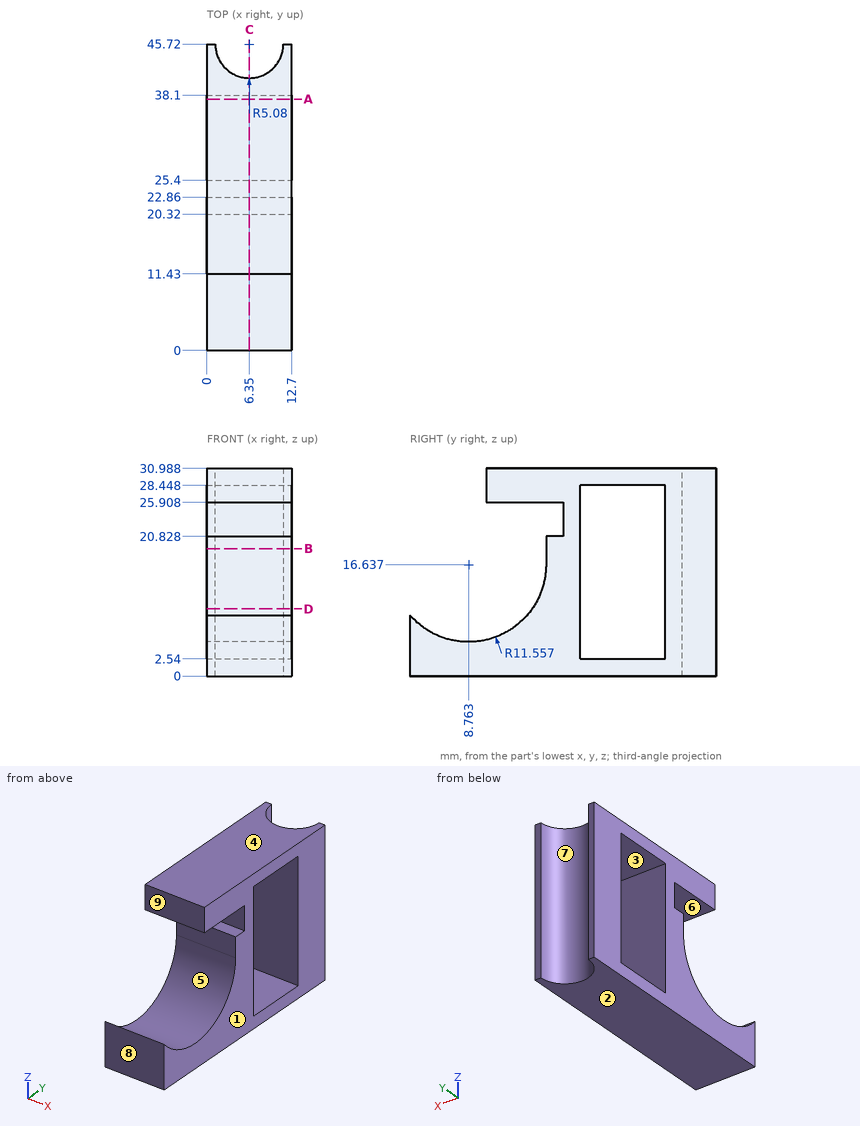
For this review, use the dimensioned drawing (mm, ordinates from the lowest corner) and the shaded views. A direction names the side the tool comes from. Give positions to 0.01 mm unless a question says otherwise; leave off trailing zeros. Order: outer loops, then holes, each group sorted by start corner. A loop starts at its lowest first (then second) coordinate and runs counter-clockwise, first axis right, second up.
1) Wall thickness on line 1 (Z direction, x = 6.25, y = 30); line 2 (Y direction, x = 3, z = 6); line 3 (Z direction, x = 1, y = 19): over which ranges is each line inside the solid? List them lowest first.
2) Take a section at D-D (z = 10). Give the boundary of the cut face in (x, y), then the cut area to 3 significant figures.
3) Take a section at C-C (x = 6.35). Give the boundary of the cut face in (y, z), then the cut area to 3 significant figures.
4) Take a section at B-B (z = 19). Give the boundary of the cut face in (x, y).
5) Insertion check: pin 1 (2 mm diameter, centred on x = 5, z = 13.5, fed in from +Y); pin 2 (1.5 mm diameter, centred on x = 4, z = 22.5, fed in from -Y); pin 3 (2 mm diameter, centred on x = 10, z = 26, fed in from -Y). Each pin has a flat end and moves straight along its axis. Give the tip position at first contact, or say it passes through.
6) The part is to be moulded in two halves that separate along Z. For the marked faces 1, 2, 3 and 4, say which applies: released by +Z, released by -Z, zero draft, split by the parting line, or undercut.
7) For the marked faces 5, 6, 7, 8 and 9, list the 3-axis set-ups (+Z, -Z, +X, -X, +Y, -Y) from which the entire face can be reached by the end or side of a thin tool; tool diameter is ignored.
8) Take a section at A-A (y = 37.5). Give the boundary of the cut face in (x, z), then the cut area to 3 significant figures.
Derived:
1. line 1: z = 0 to 2.54, 28.45 to 30.99
1. line 2: y = 0 to 4.24, 13.28 to 25.4, 38.1 to 41.9
1. line 3: z = 0 to 11.27, 25.91 to 30.99
2. outline: (0, 18.22) - (12.7, 18.22) - (12.7, 25.4) - (0, 25.4) - close; (0, 38.1) - (12.7, 38.1) - (12.7, 45.72) - (11.43, 45.72) arc R5.08 cw to (1.27, 45.72) - (0, 45.72) - close
2. area: 147 mm2
3. outline: (0, 0) - (40.64, 0) - (40.64, 30.99) - (11.43, 30.99) - (11.43, 25.91) - (22.86, 25.91) - (22.86, 20.83) - (20.32, 20.83) - (20.32, 16.64) arc R11.56 cw to (0, 9.1) - close; hole (25.4, 2.54) - (38.1, 2.54) - (38.1, 28.45) - (25.4, 28.45) - close
3. area: 476 mm2
4. outline: (0, 20.32) - (12.7, 20.32) - (12.7, 25.4) - (0, 25.4) - close; (0, 38.1) - (12.7, 38.1) - (12.7, 45.72) - (11.43, 45.72) arc R5.08 cw to (1.27, 45.72) - (0, 45.72) - close
5. pin 1: stops at y = 41.22
5. pin 2: stops at y = 22.86
5. pin 3: stops at y = 11.43
6. face 1: zero draft
6. face 2: released by -Z
6. face 3: undercut
6. face 4: released by +Z
7. face 5: +X, -X
7. face 6: +X, -X, -Y
7. face 7: +Z, -Z, +Y
7. face 8: +Z, -Z, +X, -X, -Y
7. face 9: +Z, +X, -X, -Y
8. outline: (0, 0) - (12.7, 0) - (12.7, 2.54) - (0, 2.54) - close; (0, 28.45) - (12.7, 28.45) - (12.7, 30.99) - (0, 30.99) - close
8. area: 64.5 mm2
